Input: part model. Units: mm. Frame: model coordinates. Give positions to 0.01 mm unless a question says otherwise; leave off trailing zeros. Write each loop counter-clockwise with the first axis right and the second up, starting at its lowest first coordinate (ties: lowest second). Pieces come first, ordered by that corner, then holes. Notation, with made-up numbers: (60, 33) - (75, 33) arc R23 ccw to (75, 60) - close; hole circle Ø8 at (6.25, 49.5). An arc over 180 degrees is marked (long way). Answer as CSV lines item,"result".
Autodesk Inventor part; units mm, degrees
ref_plane "YZ Plane" through (0, 0, 0) normal (1, 0, 0) x (0, 1, 0)
ref_plane "XZ Plane" through (0, 0, 0) normal (0, 1, 0) x (-1, 0, 0)
ref_plane "XY Plane" through (0, 0, 0) normal (0, 0, 1) x (1, 0, 0)
sketch "Náčrt1" plane through (0, 0, 0) normal (0, 0, 1) x (1, 0, 0)
  line L0 (0, 0) -> (-25, 0) construction
  line L1 (-25, 0) -> (-25, -14) construction
  line L2 (-25, -14) -> (0, -14) construction
  line L3 (0, -14) -> (0, 0) construction
  line L4 (-25, -14) -> (25, -14)
  line L5 (25, -14) -> (25, 14)
  line L6 (25, 14) -> (-25, 14)
  line L7 (-25, 14) -> (-25, -14)
  dimension "d0" = 25
  dimension "d1" = 14
  dimension "d2" = 50
  dimension "d3" = 28
extrude "Vysunutí1" add sketch "Náčrt1" along normal blind 14
fillet "Zaoblení1" radius 5 4 edges at (0, 14, 14) (0, 14, 0) (0, -14, 14) (0, -14, 0)
properties part number "7.4 V  500MaH Li pol"
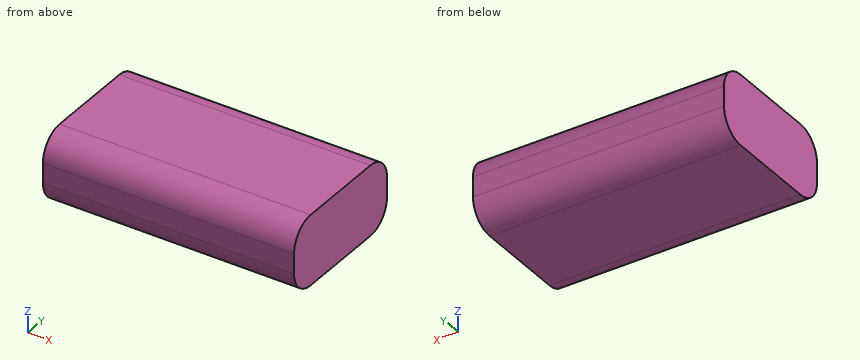
Item 1: Cut plane C-C on z = 1.75. Return the cut outline in (x, y), plus the area to 3 significant figures.
The answers:
outline,"(-25, -12.8) - (25, -12.8) - (25, 12.8) - (-25, 12.8) - close"
area,"1,280 mm²"
Item 2: Cut plane B-B on y = 12. Return the cut outline in (x, z).
The answers:
outline,"(-25, 1) - (25, 1) - (25, 13) - (-25, 13) - close"
Item 3: Contact query for a flat-ended pin moving along its axis: pin 1 (8 mm diameter, centred on x = 4.5, y = 8.5, fed in from -Z). Output: stop coordinate, or through.
The answers:
pin 1,"z = 0"
Item 4: Ray query, line 1 (Y direction, x = 12.5, z = 11); line 2 (Z direction, x = 2, y = 10); line 3 (Z direction, x = 23, y = 10.25). Return the intervals inside material, ascending. Write a range as from..to.
The answers:
line 1,"-13.58..13.58"
line 2,"0.1..13.9"
line 3,"0.16..13.84"
Item 5: Cut plane A-A on x = -13. Return the cut outline in (y, z), plus the area to 3 significant figures.
The answers:
outline,"(-14, 5) arc R5 ccw to (-9, 0) - (9, 0) arc R5 ccw to (14, 5) - (14, 9) arc R5 ccw to (9, 14) - (-9, 14) arc R5 ccw to (-14, 9) - close"
area,"371 mm²"
